Answer from the drawing. Dimensions are ordinates in mm from the lowest x, y and z of the part. A direction names the side the tool comes from. Give positions to 0.01 mm unless a question says otherwise; leave off trailing zeros. Write each loop counter-clockwise with the first axis right and the second up, starting at its lowest first coordinate (ties: lowest second). Pieces come first, ordered by that corner, then holes. Notation, with made-up numbers: (60.5, 89) -> (113.5, 89) arc R28 ccw to (113.5, 115) -> close; hole circle Ø4 at (41.5, 70.25). An arc over 180 degrees is marked (long way). Write item = value, one per line.
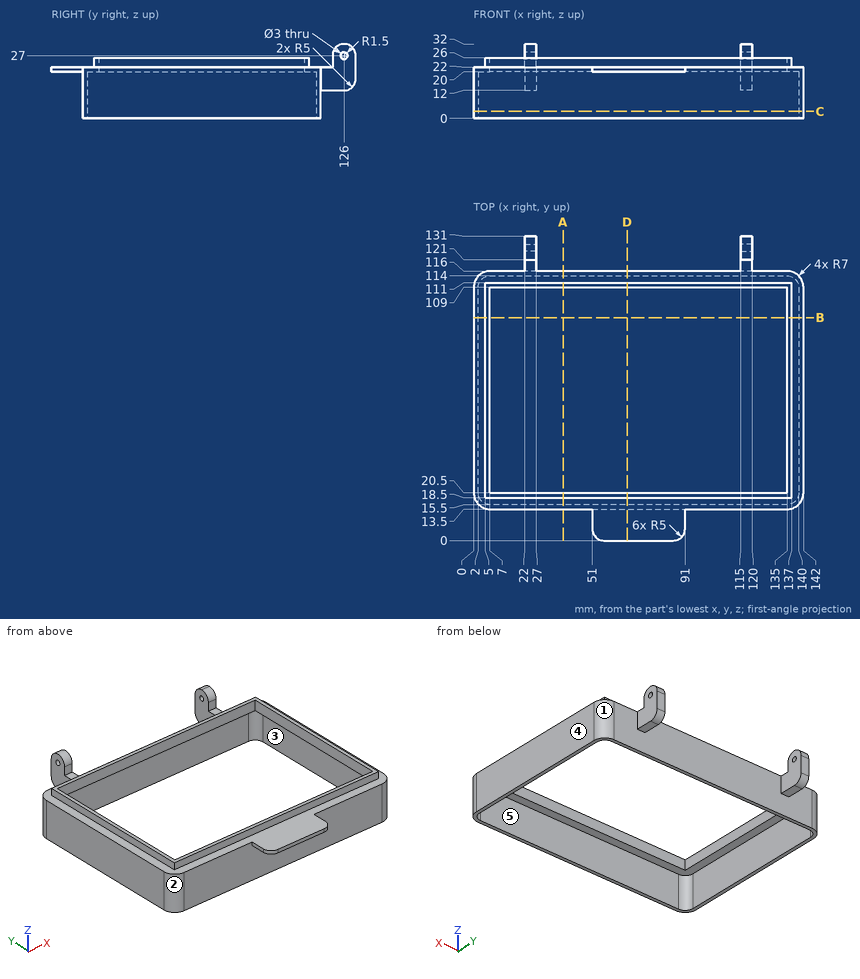
(1) Given P1, Ø3, axis at x = 73, z = 5.5, coming from the -Y side; P2, Ø7.5, axis at y = 120, z = 19, coming from the -X side; P3, Ø1.8, axis at x = 88, z = 23.5, coming from the -Y side; P4, Ø10, axis at x = 122, y = 30, coming from the +Z side, each flat-ended and moving along its own axis, determine where each tip first touches the part or whether it passes through.
Checks:
P1 = 13.5
P2 = 22
P3 = 18.5
P4 = through
(2) The part is cut by section D-D on x = 66. Determine the outline of the cut face in (y, z), plus the area to 3 significant figures.
Checks:
outline = (0, 20) -> (13.5, 20) -> (13.5, 0) -> (15.5, 0) -> (15.5, 20) -> (20.5, 20) -> (20.5, 26) -> (18.5, 26) -> (18.5, 22) -> (0, 22) -> close; (109, 20) -> (114, 20) -> (114, 0) -> (116, 0) -> (116, 22) -> (111, 22) -> (111, 26) -> (109, 26) -> close
area = 151 mm²
(3) Consider L1, parallel to X at y = 38, z = 24.5; L2, parallel to X at y = 50, z = 17.5; L3, parallel to Y at x = 48, z = 7. Determine where each line is inside the solid, lowest interval first.
Checks:
L1 = 5 to 7, 135 to 137
L2 = 0 to 2, 140 to 142
L3 = 13.5 to 15.5, 114 to 116
(4) The part is cut by section C-C on z = 3. Determine the outline of the cut face in (x, y), plus the area to 3 significant figures.
Checks:
outline = (0, 20.5) arc R7 ccw to (7, 13.5) -> (135, 13.5) arc R7 ccw to (142, 20.5) -> (142, 109) arc R7 ccw to (135, 116) -> (7, 116) arc R7 ccw to (0, 109) -> close; hole (2, 20.5) arc R5 ccw to (7, 15.5) -> (135, 15.5) arc R5 ccw to (140, 20.5) -> (140, 109) arc R5 ccw to (135, 114) -> (7, 114) arc R5 ccw to (2, 109) -> close
area = 941 mm²
(5) For a pull along Y with two mould halves and no side action, classify the marked faces 1, 2 and 3 as released by +Y, released by -Y, zero draft, split by the parting line, or undercut.
Checks:
face_1 = released by +Y
face_2 = released by -Y
face_3 = undercut
(6) The part is cut by section B-B on y = 96. Determine the outline of the cut face in (x, z).
Checks:
outline = (0, 0) -> (2, 0) -> (2, 20) -> (7, 20) -> (7, 26) -> (5, 26) -> (5, 22) -> (0, 22) -> close; (135, 20) -> (140, 20) -> (140, 0) -> (142, 0) -> (142, 22) -> (137, 22) -> (137, 26) -> (135, 26) -> close
(7) The part is cut by section A-A on x = 38.5. Determine the outline of the cut face in (y, z), plus the area to 3 significant figures.
Checks:
outline = (13.5, 0) -> (15.5, 0) -> (15.5, 20) -> (20.5, 20) -> (20.5, 26) -> (18.5, 26) -> (18.5, 22) -> (13.5, 22) -> close; (109, 20) -> (114, 20) -> (114, 0) -> (116, 0) -> (116, 22) -> (111, 22) -> (111, 26) -> (109, 26) -> close
area = 124 mm²
(8) A tool of negligible diameter and unlimited length cuts with its end or side. For the marked faces 4 and 5, from which of +Z, -Z, +X, -X, +Y, -Y can it reach the whole face along a straight path? Write none if from no direction.
Checks:
face_4 = +Z, -Z, +X, +Y, -Y
face_5 = -Z
